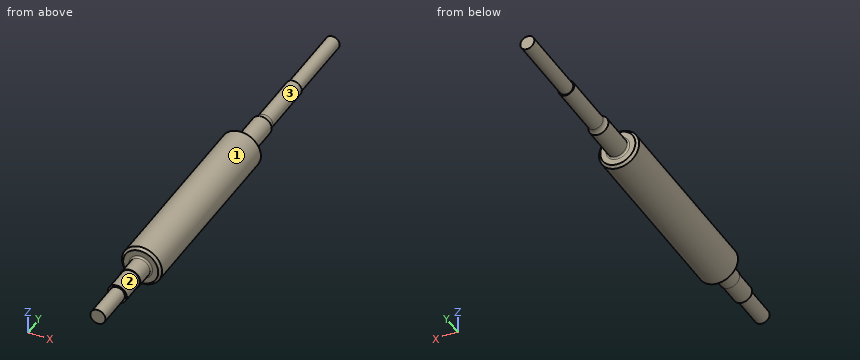
from build123d import *

# Parameters (mm, degrees)
SKETCH1_R           = 7.975
BOSS_EXTRUDE1_DEPTH = 78.2
SKETCH2_R           = 4
BOSS_EXTRUDE2_DEPTH = 15
BOSS_EXTRUDE3_START = 8
SKETCH3_R           = 4
BOSS_EXTRUDE3_DEPTH = 8
SKETCH4_R           = 3.195
BOSS_EXTRUDE4_DEPTH = 24.7
SKETCH5_R           = 2.79
BOSS_EXTRUDE5_DEPTH = 30
BOSS_EXTRUDE7_START = 8
SKETCH3_2_R         = 4
BOSS_EXTRUDE7_DEPTH = 8
SKETCH11_R          = 3.76
BOSS_EXTRUDE8_DEPTH = 10
SKETCH12_R          = 3
BOSS_EXTRUDE9_DEPTH = 15
CHAMFER6_SIZE       = 1
CHAMFER7_SIZE       = 1
FILLET1_R           = 0.7
FILLET3_R           = 0.7
FILLET4_R           = 4


with BuildPart() as part:
    # Sketch1 → Boss-Extrude1 (new body)
    with BuildSketch(Plane(origin=(0, 0, 0), x_dir=(1, 0, 0), z_dir=(0, 1, 0))):
        with Locations(Location((0, 0, 0), (0, 0, 270))):
            Circle(SKETCH1_R)
    extrude(amount=BOSS_EXTRUDE1_DEPTH)

    # Sketch2 → Boss-Extrude2 (add)
    with BuildSketch(Plane(origin=(0, 78.2, 0), x_dir=(1, 0, 0), z_dir=(0, 1, 0))):
        with Locations(Location((0, 0, 0), (0, 0, 270))):
            Circle(SKETCH2_R)
    extrude(amount=BOSS_EXTRUDE2_DEPTH)

    # Sketch3 → Boss-Extrude3 (add)
    with BuildSketch(Plane.XZ.offset(BOSS_EXTRUDE3_START)):
        with Locations(Location((0, 0, 0), (0, 0, 90))):
            Circle(SKETCH3_R)
    extrude(amount=-BOSS_EXTRUDE3_DEPTH)

    # Sketch4 → Boss-Extrude4 (add)
    with BuildSketch(Plane(origin=(0, 93.2, 0), x_dir=(1, 0, 0), z_dir=(0, 1, 0))):
        with Locations(Location((0, 0, 0), (0, 0, 270))):
            Circle(SKETCH4_R)
    extrude(amount=BOSS_EXTRUDE4_DEPTH)

    # Sketch5 → Boss-Extrude5 (add)
    with BuildSketch(Plane(origin=(0, 117.9, 0), x_dir=(1, 0, 0), z_dir=(0, 1, 0))):
        with Locations(Location((0, 0, 0), (0, 0, 270))):
            Circle(SKETCH5_R)
    extrude(amount=BOSS_EXTRUDE5_DEPTH)

    # Sketch3<2> → Boss-Extrude7 (add)
    with BuildSketch(Plane.XZ.offset(BOSS_EXTRUDE7_START)):
        with Locations(Location((0, 0, 0), (0, 0, 90))):
            Circle(SKETCH3_2_R)
    extrude(amount=-BOSS_EXTRUDE7_DEPTH)

    # Sketch11 → Boss-Extrude8 (add)
    with BuildSketch(Plane.XZ.offset(8)):
        with Locations(Location((0, 0, 0), (0, 0, 270))):
            Circle(SKETCH11_R)
    extrude(amount=BOSS_EXTRUDE8_DEPTH)

    # Sketch12 → Boss-Extrude9 (add)
    with BuildSketch(Plane.XZ.offset(18)):
        with Locations(Location((0, 0, 0), (0, 0, 270))):
            Circle(SKETCH12_R)
    extrude(amount=BOSS_EXTRUDE9_DEPTH)

    # Chamfer6
    chamfer6_edges = [part.edges().sort_by_distance(p)[0] for p in [
        (0, 78.2, -7.975),
    ]]
    chamfer(chamfer6_edges, length=CHAMFER6_SIZE)

    # Chamfer7
    chamfer7_edges = [part.edges().sort_by_distance(p)[0] for p in [
        (0, 0, -7.975),
    ]]
    chamfer(chamfer7_edges, length=CHAMFER7_SIZE)

    # Fillet1
    fillet1_edges = [part.edges().sort_by_distance(p)[0] for p in [
        (0, 78.2, -4),
    ]]
    fillet(fillet1_edges, radius=FILLET1_R)

    # Fillet3
    fillet3_edges = [part.edges().sort_by_distance(p)[0] for p in [
        (0, 0, -4),
    ]]
    fillet(fillet3_edges, radius=FILLET3_R)

    # Fillet4
    # the kernel refuses this fillet: 4 mm, written as the material it adds along each edge
    with BuildSketch(Plane(origin=(0, 93.2, 0), x_dir=(0, 0, 1), z_dir=(-1, 0, 0))) as fillet4_piece_1:
        with BuildLine():
            CenterArc((7.195, 2.406652239), FILLET4_R, 180, 36.989098612)
            Line((3.195, 2.406652239), (3.115, 2.406652239))
            Line((3.115, 2.406652239), (3.115, 0))
            Line((3.115, 0), (3.195, -0.08))
            ThreePointArc((3.195, -0.08), (3.5975, -0.08), (3.9361, -0.048133045))
            Line((3.9361, -0.048133045), (4, 0))
        make_face()
    revolve(axis=Axis((0, 93.2, 0), (0, 1, 0)))


solid = part.part
Build history of the part. All positions in model axes, mm. Face numbers are marked on the shaded views. A direction names the side the tool comes from. Coordinates: 2 decimals unless noted, no trailing zeros. Write each loop counter-clockwise with the first axis right and the second up, starting at its lowest first coordinate (ties: lowest second). Pieces come first, ordered by that corner, then holes.
(1) Drill centre lines: line 1 (X direction, y = 43, z = -0.75); line 2 (Y direction, x = -2.75, z = -1.5); line 3 (Y direction, x = 3, z = -3.5). Where is each one in solid material? Low to high.
(2) Cut at A-A on y = 33.5. List the corners of the cut face in (x, z) (3 decimals), and give its area (3 significant figures).
(3) Pin check, flat tips, straight feed: pin 1 Ø1.5 at (x, z) = (-6.5, 0) entering from -Y; pin 2 Ø6 at (x, y) = (-4.5, 35.5) entering from +Z; pin 3 Ø2 at (y, z) = (66, -2) entering from +X. Stop position of each tip, or through.
(4) 3-axis set-ups, long thin cutter, end or side, ignore diameter. For the marked faces 1, 2 and 3: which of +Z, -Z, +X, -X, +Y, -Y reach the whole face in a straight line?
(5) Cut at B-B on y = 90.5. List the corners of the cut face in (x, z), and give its area (3 significant figures).
Working result:
1. line 1: x = -7.94 to 7.94
1. line 2: y = -18 to 117.9
1. line 3: y = -0.01 to 78.21
2. outline: circle Ø15.95 at (0, 0)
2. area: 200 mm2
3. pin 1: stops at y = 0
3. pin 2: stops at z = 7.83
3. pin 3: stops at x = 7.91
4. face 1: +Y, -Y
4. face 2: -Y
4. face 3: +Y
5. outline: circle Ø8 at (0, 0)
5. area: 50.3 mm2
